from build123d import *

# Parameters (mm, degrees)
SKETCH1_R           = 2.5
BOSS_EXTRUDE1_DEPTH = 5


with BuildPart() as part:
    # Sketch1 → Boss-Extrude1 (new body)
    with BuildSketch(Plane(origin=(0, 0, 0), x_dir=(1, 0, 0), z_dir=(0, 1, 0))):
        with BuildLine():
            Line((25, -50), (40, -50))
            ThreePointArc((40, -50), (47.071067812, -47.071067812), (50, -40))
            Line((50, -40), (50, -25))
            Line((50, -25), (40, -25))
            Line((40, -25), (40, -15))
            Line((40, -15), (50, -15))
            Line((50, -15), (50, 15))
            Line((50, 15), (40, 15))
            Line((40, 15), (40, 25))
            Line((40, 25), (50, 25))
            Line((50, 25), (50, 40))
            ThreePointArc((50, 40), (47.071067812, 47.071067812), (40, 50))
            Line((40, 50), (30, 50))
            Line((30, 50), (25, 50))
            Line((25, 50), (25, 40))
            Line((25, 40), (15, 40))
            Line((15, 40), (15, 50))
            Line((15, 50), (-15, 50))
            Line((-15, 50), (-15, 40))
            Line((-15, 40), (-25, 40))
            Line((-25, 40), (-25, 50))
            Line((-25, 50), (-40, 50))
            ThreePointArc((-40, 50), (-47.071067812, 47.071067812), (-50, 40))
            Line((-50, 40), (-50, 25))
            Line((-50, 25), (-40, 25))
            Line((-40, 25), (-40, 15))
            Line((-40, 15), (-50, 15))
            Line((-50, 15), (-50, -15))
            Line((-50, -15), (-40, -15))
            Line((-40, -15), (-40, -25))
            Line((-40, -25), (-50, -25))
            Line((-50, -25), (-50, -40))
            ThreePointArc((-50, -40), (-47.071067812, -47.071067812), (-40, -50))
            Line((-40, -50), (-25, -50))
            Line((-25, -50), (-25, -40))
            Line((-25, -40), (-15, -40))
            Line((-15, -40), (-15, -50))
            Line((-15, -50), (15, -50))
            Line((15, -50), (15, -40))
            Line((15, -40), (25, -40))
            Line((25, -40), (25, -50))
        make_face()
        with Locations((-30, -45)):
            Circle(SKETCH1_R, mode=Mode.SUBTRACT)
        with Locations((-45, -30)):
            Circle(SKETCH1_R, mode=Mode.SUBTRACT)
        with Locations((30, -45)):
            Circle(SKETCH1_R, mode=Mode.SUBTRACT)
        with Locations((45, -30)):
            Circle(SKETCH1_R, mode=Mode.SUBTRACT)
        with Locations((-45, 30)):
            Circle(SKETCH1_R, mode=Mode.SUBTRACT)
        with Locations((-30, 45)):
            Circle(SKETCH1_R, mode=Mode.SUBTRACT)
        with Locations((45, 30)):
            Circle(SKETCH1_R, mode=Mode.SUBTRACT)
        with Locations((30, 45)):
            Circle(SKETCH1_R, mode=Mode.SUBTRACT)
    extrude(amount=BOSS_EXTRUDE1_DEPTH)


solid = part.part
Geometry: final body of the model. Coordinates: model frame, mm. A direction names the side the tool comes from. Coordinates: 2 decimals unless noted, no trailing zeros. Order: outer loops, then holes, each group sorted by start corner. A loop starts at its lowest first (then second) coordinate and runs counter-clockwise, first axis right, second up.
(1) Section query C-C (z = -45). Return the cut outline in (x, y).
(2) Section query D-D (y = 3.7). State how many separate pieces and enclosed holes the cut face has, plus the area to 3 significant figures.
(3) Draft query along Z for faces 1 (the face through (46.99, 2.46, 47.15)), 2 (the face through (45, 2, 15)), 3 (the face through (-45, 2, -25)), 4 (the face through (50, 2, 0)). Return one class per face: pulls with the +Z half, pulls with the -Z half, needs draft (parallel to the pull), parting line crosses it, or undercut.
(4) Section query B-B (z = 30). Return the cut outline in (x, y), plus the area to 3 significant figures.
(5) Material intervals for probe 1 along X at (y, z) = (1.8, 30); probe 2 along Z at (x, y) = (40.5, 3.95), sorted ascending.
(6) Section query A-A (x = -30). Return the cut outline in (y, z), plus the area to 3 significant figures.
(7) Access query for faces 5 (the face through (-33, 2, 50)), 6 (the face through (-45, 2, -15)), 7 (the face through (45, 2, 25)), 8 (the face through (-15, 2, -45)). Directions: +Z, -Z, +X, -X, +Y, -Y. A direction counts if a zero-diameter tool reaches every point of the face in a straight line with its end or side. Return the directions, or none.
(8) First-contact query: pin 1 (4.5 mm diameter, centred on x = -45, z = -30, fed in from +Y); pin 2 (6 mm diameter, centred on x = 45, z = 30, fed in from -Y); pin 3 (1.5 mm diameter, centred on y = 2, z = 43.5, fed in from +X); pin 4 (2.5 mm diameter, centred on y = 3, z = 22, fed in from -X). Flat tips, straight axial feed; report the tip coordinate or a pass-through.
Solution:
1. outline: (-48.66, 0) - (-32.5, 0) - (-32.5, 5) - (-48.66, 5) - close; (-27.5, 0) - (-25, 0) - (-25, 5) - (-27.5, 5) - close; (-15, 0) - (15, 0) - (15, 5) - (-15, 5) - close; (25, 0) - (27.5, 0) - (27.5, 5) - (25, 5) - close; (32.5, 0) - (48.66, 0) - (48.66, 5) - (32.5, 5) - close
2. separate pieces: 1
2. enclosed holes: 8
2. area: 8,960 mm2
3. face 1: pulls with the +Z half
3. face 2: undercut
3. face 3: undercut
3. face 4: needs draft
4. outline: (-50, 0) - (-47.5, 0) - (-47.5, 5) - (-50, 5) - close; (-42.5, 0) - (42.5, 0) - (42.5, 5) - (-42.5, 5) - close; (47.5, 0) - (50, 0) - (50, 5) - (47.5, 5) - close
4. area: 450 mm2
5. probe 1: x = -50 to -47.5, -42.5 to 42.5, 47.5 to 50
5. probe 2: z = -49.99 to -25, -15 to 15, 25 to 49.99
6. outline: (0, -50) - (5, -50) - (5, -47.5) - (0, -47.5) - close; (0, -42.5) - (5, -42.5) - (5, 42.5) - (0, 42.5) - close; (0, 47.5) - (5, 47.5) - (5, 50) - (0, 50) - close
6. area: 450 mm2
7. face 5: +Z, +X, -X, +Y, -Y
7. face 6: -X, +Y, -Y
7. face 7: +X, +Y, -Y
7. face 8: -Z, +Y, -Y
8. pin 1: passes through
8. pin 2: stops at y = 0
8. pin 3: stops at x = 49.61
8. pin 4: stops at x = -40
